Model file for the job. Use its own axes, mm. Face numbers are marked on the shaded views. A direction names the side the tool comes from. Give positions to 0.01 mm unless a question says otherwise; leave off trailing zeros. Order: outer loops, then holes, each group sorted by start corner. A loop starts at its lowest first (then second) coordinate and runs counter-clockwise, first axis right, second up. Notation, with made-up numbers: M 34,26.5 L 87,26.5 A16 ccw 87,37.5 Z; hole C 27,0 d2. An arc over 180 degrees is marked long. Return JSON: item names as keys, results as strings. Group by question number.
1. Wall check: probe 1 along Z at (x, y) = (6.25, -8.25); probe 2 along Y at (x, z) = (18.5, 14). Give the ranges that are in metal, low to high. Write a range as [from, to].
2. Two-plate mould, pull along Z, no slides. Class the marked faces 1, 2 and 3: released by +Z, released by -Z, zero draft, split by the parting line, or undercut.
3. 3-axis set-ups, long thin cutter, end or side, ignore diameter. For the marked faces 4 and 5: which of +Z, -Z, +X, -X, +Y, -Y reach the whole face in a straight line?
4. Slice it at D-D on z = 68. List the corners of the cut face in (x, y), then the cut area to 3 significant figures.
5. Pin check, flat tips, straight feed: pin 1 (1 mm diameter, centred on x = 10, z = 95.5, fed in from -Y); pin 2 (5 mm diameter, centred on x = 4.5, z = 116.5, fed in from -Y). Stop position of each tip, or through.
6. Slice it at C-C on x = 3.25. List the corners of the cut face in (y, z), then the cut area to 4 significant figures.
7. Slice it at B-B on x = 12.5. Give the number of separate pieces and of enclosed holes in the cut face, then the cut area to 3 significant figures.
8. Slice it at A-A on y = -6.25. List the corners of the cut face in (x, z), then the cut area to 3 significant figures.
from build123d import *

# Parameters (mm, degrees)
ESQUISSE1_W             = 30
ESQUISSE1_H             = 10
BOSS_EXTRU_1_DEPTH      = 130.5
ESQUISSE2_W             = 30
ESQUISSE2_H             = 5
BOSS_EXTRU_2_DEPTH      = 20
ESQUISSE3_R             = 3.15
ENL_V_MAT_EXTRU_2_DEPTH = 136.389253636


with BuildPart() as part:
    # Esquisse1 → Boss.-Extru.1 (new body)
    with BuildSketch(Plane.XY):
        with Locations((15, 5)):
            Rectangle(ESQUISSE1_W, ESQUISSE1_H)
    extrude(amount=BOSS_EXTRU_1_DEPTH)

    # Esquisse2 → Boss.-Extru.2 (add)
    with BuildSketch(Plane.XZ):
        with Locations((15, 2.5)):
            Rectangle(ESQUISSE2_W, ESQUISSE2_H)
        with Locations((15, 18)):
            Rectangle(ESQUISSE2_W, ESQUISSE2_H)
        with Locations((15, 128)):
            Rectangle(ESQUISSE2_W, ESQUISSE2_H)
        with Locations((15, 112.5)):
            Rectangle(ESQUISSE2_W, ESQUISSE2_H)
    extrude(amount=BOSS_EXTRU_2_DEPTH)

    # Esquisse3 → Enlèv. mat.-Extru.2 (cut, through all)
    with BuildSketch(Plane.XY.offset(130.5)):
        with Locations((14.302143115, -10.686909811)):
            Circle(ESQUISSE3_R)
    extrude(amount=-ENL_V_MAT_EXTRU_2_DEPTH, mode=Mode.SUBTRACT)


solid = part.part
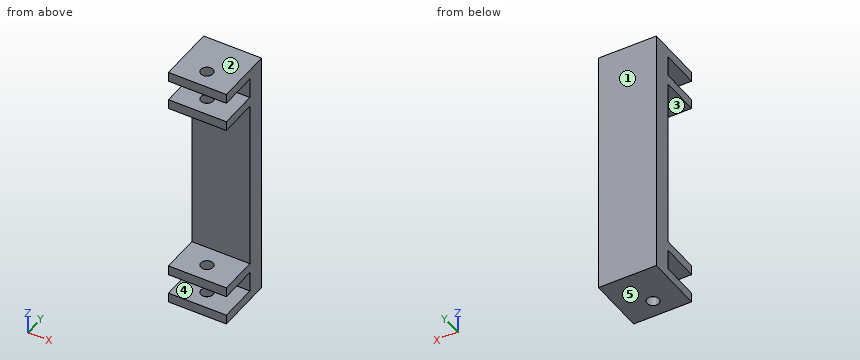
Result:
{
 "1": {"probe 1": "z = [0, 5], [15.5, 20.5], [110, 115], [125.5, 130.5]", "probe 2": "y = [0, 10]"},
 "2": {"face 1": "zero draft", "face 2": "released by +Z", "face 3": "undercut"},
 "3": {"face 4": "+X, -X, -Y", "face 5": "-Z, +X, -X, +Y, -Y"},
 "4": {"outline": "M 0,0 L 30,0 L 30,10 L 0,10 Z", "area": "300 mm2"},
 "5": {"pin 1": "stops at y = 0", "pin 2": "stops at y = -20"},
 "6": {"outline": "M -20,0 L 10,0 L 10,130.5 L -20,130.5 L -20,125.5 L 0,125.5 L 0,115 L -20,115 L -20,110 L 0,110 L 0,20.5 L -20,20.5 L -20,15.5 L 0,15.5 L 0,5 L -20,5 Z", "area": "1,705 mm2"},
 "7": {"separate pieces": "5", "enclosed holes": "0", "area": "1,600 mm2"},
 "8": {"outline": "M 0,0 L 30,0 L 30,5 L 0,5 Z; M 0,15.5 L 30,15.5 L 30,20.5 L 0,20.5 Z; M 0,110 L 30,110 L 30,115 L 0,115 Z; M 0,125.5 L 30,125.5 L 30,130.5 L 0,130.5 Z", "area": "600 mm2"}
}
